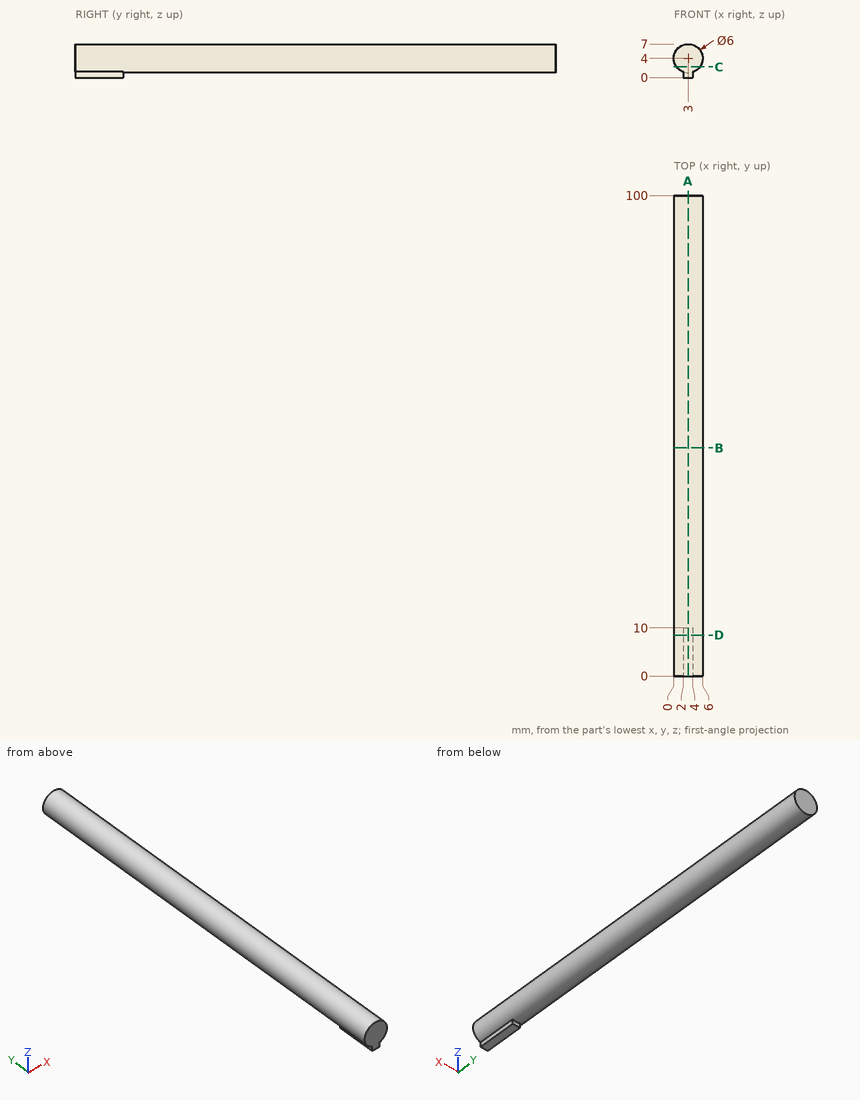
Source: three-view drawing plus pictorial views. Frame: mm from the lowest corner of the part. Coordinates: 2 decimals unless noted, no trailing zeros. Loops run counter-clockwise (first coordinate to the right, second up) from the corner with the lowest first, then second, coordinate; pieces in that order, holes last. Notation, with made-up numbers: M 49.5,-19 L 55.5,-19 A26 ccw 55.5,14 Z; hole C -2.75,2 d6. An arc over 180 degrees is marked long. Use CSV: the item, a comma, the result in double quotes.
(1) Cut plane A-A on x = 3. Return loops of the section in (y, z), and give its area (3 significant figures).
Answers follow:
outline,"M 0,0 L 10,0 L 10,1 L 100,1 L 100,7 L 0,7 Z"
area,"610 mm²"
(2) Cut plane B-B on y = 47.5. Return loops of the section in (x, z).
Answers follow:
outline,"C 3,4 d6"
(3) Cut plane C-C on z = 2.25. Return loops of the section in (x, y), and give its area (3 significant figures).
Answers follow:
outline,"M 0.56,0 L 5.44,0 L 5.44,100 L 0.56,100 Z"
area,"487 mm²"
(4) Line query: line 1 (Y direction, x = 2.95, z = 0.5); line 2 (X direction, y = 16, z = 6.25); line 3 (Z direction, x = 1.2, y = 23). Output: solid intervals per line, ascending. Write a range as [from, to].
Answers follow:
line 1,"[0, 10]"
line 2,"[1.02, 4.98]"
line 3,"[1.6, 6.4]"
(5) Cut plane D-D on y = 8.5. Return loops of the section in (x, z), and give its area (3 significant figures).
Answers follow:
outline,"M 2,0 L 4,0 L 4,1.17 A3 ccw long 2,1.17 Z"
area,"30.4 mm²"
(6) Contact query for flat-ended pins moving along their axis: pin 1 (1 mm diameter, centred on x = 1.5, y = 26, fed in from +Z); pin 2 (0.6 mm diameter, centred on y = 3.5, z = 0.5, fed in from +X); pin 3 (0.6 mm diameter, centred on x = 3, z = 0.5, fed in from +Y). Output: stop coordinate, or through.
Answers follow:
pin 1,"z = 6.83"
pin 2,"x = 4"
pin 3,"y = 10"
